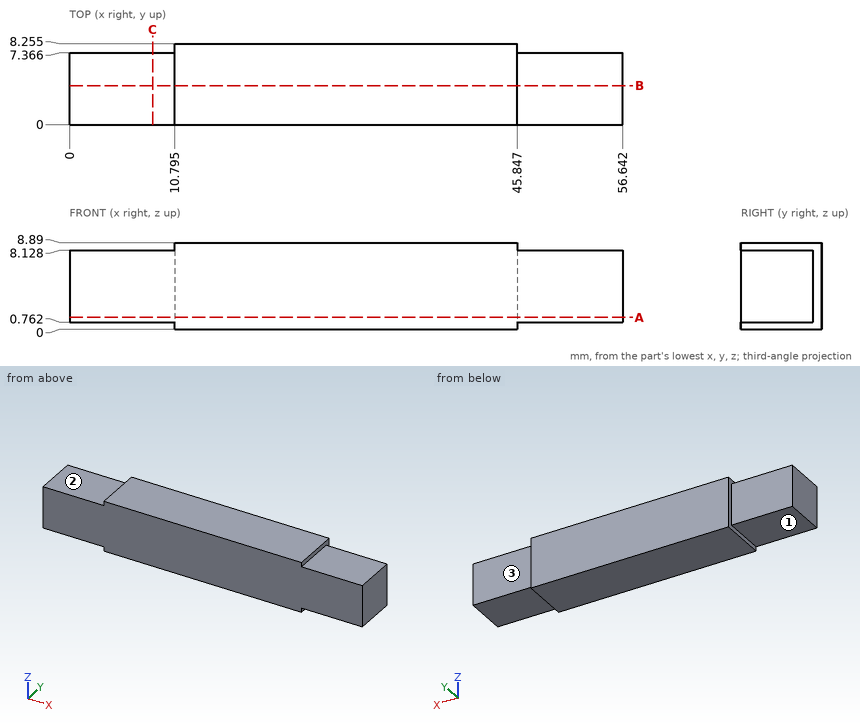
Design review of the part shown in the three views and the two pictorial views. Dimensions are in mm from the part's minimum x, y and z. A direction names the side the tool comes from. Round coordinates to 2 decimals unless told otherwise and drop trailing zeros. Loops run counter-clockwise (first coordinate to the right, second up) from the corner with the lowest first, then second, coordinate; pieces in that order, holes last. Notation, with made-up numbers: (-18, 3) -> (7, 3) arc R18 ccw to (7, 14) -> close; hole circle Ø6 at (-12.5, -10.5). An arc over 180 degrees is marked (long way). Return JSON: item names as keys, results as strings.
(1) Add section B-B on y = 4. Write out the cut boundary in (x, z) (3 decimals), plus the area to 3 significant figures.
Solved:
{"outline": "(0, 0.762) -> (10.795, 0.762) -> (10.795, 0) -> (45.847, 0) -> (45.847, 0.762) -> (56.642, 0.762) -> (56.642, 8.128) -> (45.847, 8.128) -> (45.847, 8.89) -> (10.795, 8.89) -> (10.795, 8.128) -> (0, 8.128) -> close", "area": "471 mm2"}
(2) For line 1 (X direction, y = 7.5, z = 2.25) (3 decimals); line 2 (Y direction, x = 9.5, z = 1.75); line 3 (Z direction, x = 53, y = 5.5), list the stretches that pass through material, from the lowest coordinate up.
Solved:
{"line 1": "10.795 to 45.847", "line 2": "0 to 7.37", "line 3": "0.76 to 8.13"}
(3) For pin 1 (1 mm diameter, centred on x = 47.5, z = 4.5, fed in from +Y); pin 2 (2 mm diameter, centred on x = 52, y = 4.5, fed in from +Z); pin 3 (1.5 mm diameter, centred on x = 7.5, y = 2.5, fed in from -Z), all flat-tipped, find the tip position at first contact; note any pin that passes through.
Solved:
{"pin 1": "y = 7.37", "pin 2": "z = 8.13", "pin 3": "z = 0.76"}
(4) Add section C-C on x = 8.5. Write out the cut boundary in (y, z), plus the area to 3 significant figures.
Solved:
{"outline": "(0, 0.76) -> (7.37, 0.76) -> (7.37, 8.13) -> (0, 8.13) -> close", "area": "54.3 mm2"}
(5) For the marked faces 1, 2 and 3, list the 3-axis set-ups (+Z, -Z, +X, -X, +Y, -Y) from which the entire face can be reached by the end or side of a thin tool; tool diameter is ignored.
Solved:
{"face 1": "-Z, -X, +Y, -Y", "face 2": "+Z, -X, +Y, -Y", "face 3": "+Z, -Z, +X, +Y"}
(6) Add section A-A on z = 1.25. Write out the cut boundary in (x, y) (3 decimals).
Solved:
{"outline": "(0, 0) -> (56.642, 0) -> (56.642, 7.366) -> (45.847, 7.366) -> (45.847, 8.255) -> (10.795, 8.255) -> (10.795, 7.366) -> (0, 7.366) -> close"}
